Source: CAD feature listing. Evaluate the final solid. Frame: model axes, mm. Face numbers are marked on the shaded views. Round coordinates to 2 decimals unless told otherwise and drop trailing zeros. Order: outer loops, then holes, each group sorted by start corner. A loop starts at its lowest first (then second) coordinate and runs counter-clockwise, first axis right, second up. Notation, with made-up numbers: (-36, 3) - (22, 3) arc R21 ccw to (22, 14) - close; hole circle Ø9 at (-22.75, 82). An arc over 180 degrees is marked (long way). Return JSON: item names as keys, results as strings. Group by question number.
1) Ray query, line 1 (Y direction, x = -10.75, z = 95.5); line 2 (Z direction, x = -13.5, y = 37.5); line 3 (Z direction, x = -5.75, y = -7). Return the intervals inside material, ascending. Write a range as from..to.
2) Mould query, pull axis X, two halves, no side actions, for the marked faces 1, 2 and 3. Classes: pulls with the +X half, pulls with the -X half, needs draft (parallel to the pull), parting line crosses it, or undercut.
3) Section D-D, the plane z = 15. Return loops of the section in (x, y).
4) Section A-A, the plane z = 4.5. Return loops of the section in (x, y).
5) Section B-B, the plane x = -15. Return loops of the section in (y, z), plus the area to 3 significant figures.
6) Section C-C, the plane y = 5.5. Return loops of the section in (x, z).
7) Contact query for a flat-ended pin moving along its axis: P1, Ø8, axis at y = -7, z = 85, coming from the +X side. Output: stop coordinate, or through.
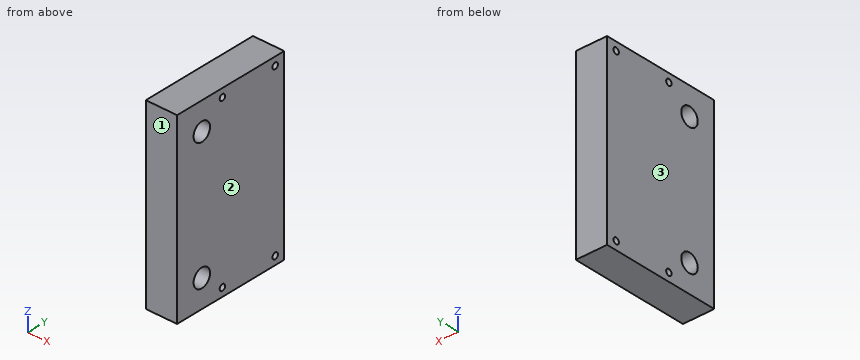
```python
from build123d import *

# Parameters (mm, degrees)
F1_DEPTH = 17
F2_D     = 3.3
F3_W     = 22
F3_H     = 100
F3_R     = 5
F4_DEPTH = 17


with BuildPart() as f1:
    # F0 (on Right) → F1 (new body)
    with BuildSketch(Plane.YZ):
        Polygon((43, 100), (0, 100), (0, 0), (43, 0), (43, 33), (43, 67), align=None)
    extrude(amount=-F1_DEPTH)

    # F2 (through all)
    with Locations(Plane.YZ):
        with Locations((37.5, 4.5), (5.5, 4.5), (5.5, 95.5), (37.5, 95.5)):
            Hole(F2_D / 2)

    # F3 (on face) → F4 (join, through all)
    with BuildSketch(Plane(origin=(-17, 0, 0), x_dir=(0, -1, 0), z_dir=(-1, 0, 0))):
        with Locations((11, 50)):
            Rectangle(F3_W, F3_H)
        with Locations((7, 15)):
            Circle(F3_R, mode=Mode.SUBTRACT)
        with Locations((7, 85)):
            Circle(F3_R, mode=Mode.SUBTRACT)
    extrude(amount=-F4_DEPTH)


solid = f1.part
```
Geometry check:
{
 "1": {"line 1": "-22..3.85, 7.15..35.85, 39.15..43", "line 2": "0..2.85, 6.15..93.85, 97.15..100", "line 3": "0..10, 20..80, 90..100"},
 "2": {"face 1": "needs draft", "face 2": "pulls with the +X half", "face 3": "pulls with the -X half"},
 "3": {"outline": "(-17, -22) - (0, -22) - (0, -12) - (-17, -12) - close; (-17, -2) - (0, -2) - (0, 43) - (-17, 43) - close"},
 "4": {"outline": "(-17, -22) - (0, -22) - (0, 3.85) - (-17, 3.85) - close; (-17, 7.15) - (0, 7.15) - (0, 35.85) - (-17, 35.85) - close; (-17, 39.15) - (0, 39.15) - (0, 43) - (-17, 43) - close"},
 "5": {"outline": "(-22, 0) - (43, 0) - (43, 100) - (-22, 100) - close; hole circle Ø10 at (-7, 15); hole circle Ø10 at (-7, 85); hole circle Ø3.3 at (5.5, 4.5); hole circle Ø3.3 at (5.5, 95.5); hole circle Ø3.3 at (37.5, 4.5); hole circle Ø3.3 at (37.5, 95.5)", "area": "6,310 mm2"},
 "6": {"outline": "(-17, 0) - (0, 0) - (0, 2.85) - (-17, 2.85) - close; (-17, 6.15) - (0, 6.15) - (0, 93.85) - (-17, 93.85) - close; (-17, 97.15) - (0, 97.15) - (0, 100) - (-17, 100) - close"},
 "7": {"P1": "through"}
}
